The listing builds one solid part. Answer for the finished solid, in the listing's coordinates (mm). A direction names the side the tool comes from. Coordinates: 2 decimals unless noted, no trailing zeros. Write each loop counter-clockwise with the first axis right and the second up, starting at its lowest first coordinate (ties: lowest second). Pieces come first, ordered by that corner, then holes. Notation, with made-up numbers: M 1,-12 L 59,-12 A20 cw 59,6 Z; hole C 26,53 d11. An arc over 180 degrees is marked long. Answer as CSV lines item,"result". Start each with the question number.
Autodesk Fusion 360 part; units mm, degrees
sketch "Sketch1" plane through (0, 0, 0) normal (0, 0, 1) x (1, 0, 0)
  circle A0 centre (0, 0) radius 10
extrude "Extrude1" add sketch "Sketch1" along normal blind 10
sketch "Sketch2" plane through (0, 0, 0) normal (0, 0, -1) x (1, 0, 0)
  circle A0 centre (0, 0) radius 10
  line L0 (0, 2.5) -> (30, 2.5)
  line L1 (30, 2.5) -> (30, -2.5)
  line L2 (30, -2.5) -> (0, -2.5)
  line L3 (0, -2.5) -> (0, 2.5)
  line L4 (0, 2.5) -> (30, -2.5) construction
  line L5 (30, 2.5) -> (0, -2.5) construction
  line L6 (15, 0) -> (0, 0) construction
  point P0 (15, 0)
  dimension "d19" = 5
  dimension "d20" = 30
extrude "Extrude2" add sketch "Sketch2" against normal up to surface (10 mm away) contours A0 L0 L1 L2
hole "Hole1" at (0, 0, 10) direction (0, 0, -1) diameter 3 end through all
fillet "Fillet1" radius 2.5 2 edges at (30, -2.5, 5) (30, 2.5, 5)
hole "Hole2" at (27.5, 0, 10) direction (0, 0, -1) diameter 2.5 end through all
sketch "Sketch4" plane through (0, 0, 0) normal (0, 0, -1) x (1, 0, 0)
  circle A0 centre (27.5, 0) radius 1.25
  circle A1 centre (0, 0) radius 1.5
  arc A2 (27.5, -2.5) -> (27.5, 2.5) centre (27.5, 0) ccw
  line L0 (27.5, 2.5) -> (9.6825, 2.5)
  arc A3 (9.6825, 2.5) -> (9.6825, -2.5) centre (0, 0) ccw
  line L1 (9.6825, -2.5) -> (27.5, -2.5)
  line L2 (1.5, 5.546) -> (23.5, 5.546)
  line L3 (23.5, 5.546) -> (23.5, -5.546)
  line L4 (23.5, -5.546) -> (1.5, -5.546)
  line L5 (1.5, -5.546) -> (1.5, 5.546)
  line L6 (1.5, 5.546) -> (23.5, -5.546) construction
  line L7 (23.5, 5.546) -> (1.5, -5.546) construction
  line L8 (12.5, 0) -> (23.5, 0) construction
  point P0 (12.5, 0)
  dimension "d35" = 4
extrude "Extrude4" add sketch "Sketch4" against normal up to surface (10 mm away) contours A3 L1 L3 L4 | L0 A3 L2 L3
sketch "Sketch6" plane through (0, 0, 10) normal (0, 0, 1) x (-1, 0, 0)
  line L0 (-23.5, 5.546) -> (-23.5, 2.5)
  line L1 (-23.5, 2.5) -> (-27.5, 2.5)
  arc A0 (-27.5, 2.5) -> (-27.5, -2.5) centre (-27.5, 0) ccw
  line L2 (-27.5, -2.5) -> (-23.5, -2.5)
  line L3 (-23.5, -2.5) -> (-23.5, -5.546)
  line L4 (-23.5, -5.546) -> (-8.3212, -5.546)
  arc A1 (-8.3212, -5.546) -> (-8.3212, 5.546) centre (0, 0) ccw
  line L5 (-8.3212, 5.546) -> (-23.5, 5.546)
  circle A2 centre (-27.5, 0) radius 1.25
  circle A3 centre (0, 0) radius 1.5
  circle A4 centre (-21, 0) radius 1
  dimension "d36" = 2.5
fillet "Fillet2" radius 1 4 edges at (23.5, 5.546, 5) (23.5, -5.546, 5) (23.5, 2.5, 5) (23.5, -2.5, 5)
hole "Hole4" at (21, 0, 10) direction (0, 0, -1) diameter 3.5 end through all counterbore diameter 5.7 counterbore depth 3.5
1) The part is cut by section D-D (x = 9). Determine the outline of the cut face in (y, z).
2) Which of the six approach directions +Z, -Z, +X, -X, +Y, -Y give full straight-line access (tool end or side, diameter ignored) to faces 5 (the face through (23, 0, 6.5)), 6 (the face through (23.5, -4, 5)), 7 (the face through (16, 5.546, 5))?
3) For a pull along Y with two mould halves and no side action, classify faces 1 (the face through (29, -2, 5)), 2 (the face through (19.265, 0.228, 3.204)), 3 (the face through (5, 0, 0)), 4 (the face through (28.72, 0.27, 4.93)) as +Y half, -Y half, draft (parallel to the pull), parting line (faces both ways), or undercut.
4) Each of these flat-tipped pins is pushed along its axis until it touches: P1, Ø3, axis at x = 4.5, z = 4, coming from the -Y side; P2, Ø0.8, axis at y = 4, z = 4.5, coming from the +X side; P3, Ø2.5, axis at x = 25.5, z = 6, coming from the -Y side. Where does it stop, or does it pass through?
5) Find the intervals of material crossed by line 1 (X direction, y = 0, z = 4); line 2 (X direction, y = 0, z = 8.55); line 3 (Y direction, x = 0, z = 3.25), in increasing order. Write a range as from..to.
6) The part is cut by section C-C (x = 21). Determine the outline of the cut face in (y, z).
7) The part is cut by section B-B (z = 5.75). Count the separate pieces of the cut face and the enclosed holes in it, then the cut area to 3 significant figures.
8) The part is cut by section A-A (x = 0). Determine the outline of the cut face in (y, z), then the cut area to 3 significant figures.
Completed:
1,outline,"M -5.55,0 L 5.55,0 L 5.55,10 L -5.55,10 Z"
2,face 5,"+Z"
2,face 6,"+Z, -Z, +X, -Y"
2,face 7,"+Z, -Z, +X, +Y"
3,face 1,"-Y half"
3,face 2,"undercut"
3,face 3,"draft"
3,face 4,"undercut"
4,P1,"y = -9.54"
4,P2,"x = 23.5"
4,P3,"y = -2.53"
5,line 1,"-10..-1.5, 1.5..19.25, 22.75..26.25, 28.75..30"
5,line 2,"-10..-1.5, 1.5..18.15, 23.85..26.25, 28.75..30"
5,line 3,"-10..-1.5, 1.5..10"
6,outline,"M -5.55,0 L -1.75,0 L -1.75,6.5 L -2.85,6.5 L -2.85,10 L -5.55,10 Z; M 1.75,0 L 5.55,0 L 5.55,10 L 2.85,10 L 2.85,6.5 L 1.75,6.5 Z"
7,separate pieces,"1"
7,enclosed holes,"3"
7,area,"478 mm²"
8,outline,"M -10,0 L -1.5,0 L -1.5,10 L -10,10 Z; M 1.5,0 L 10,0 L 10,10 L 1.5,10 Z"
8,area,"170 mm²"
